CAD build for the part. Positions are in the model's coordinates, mm. Face numbers are marked on the shaded views. A direction names the side the tool comes from. Give positions to 0.01 mm unless a question says otherwise; leave off trailing zeros. Write each loop counter-clockwise with the first axis right and the second up, starting at its lowest first coordinate (ties: lowest second). Pieces come first, ordered by that corner, then holes. Notation, with made-up numbers: (41.25, -19) - (69.25, -19) arc R18 cw to (69.25, -6) - close; hole circle Ø4 at (23, 42.25). An arc over 180 degrees is marked (long way). Answer as a JSON object with one key per item and string values.
from build123d import *

# Parameters (mm, degrees)
SKETCH2_R             = 16.002
BOSS_EXTRUDE2_DEPTH   = 5.8928
CUT_EXTRUDE1_DEPTH    = 2.9464
F_4_40_TAPPED_HOLE1_D = 2.2606
CUT_EXTRUDE2_DEPTH    = 24.384890418
SKETCH5_R             = 6.35
CUT_EXTRUDE3_DEPTH    = 1.5875


with BuildPart() as part:
    # Sketch2 → Boss-Extrude2 (new body)
    with BuildSketch(Plane(origin=(0, 0, 0), x_dir=(1, 0, 0), z_dir=(0, 1, 0))):
        with Locations(Location((0, 0, 0), (0, 0, 270))):
            Circle(SKETCH2_R)
    extrude(amount=BOSS_EXTRUDE2_DEPTH)

    # Sketch2_3 → Cut-Extrude1 (cut)
    with BuildSketch(Plane(origin=(0, 0, 0), x_dir=(1, 0, 0), z_dir=(0, 1, 0))):
        with BuildLine():
            ThreePointArc((9.017, 4.192712226), (0, 9.9441), (-9.017, 4.192712226))
            Line((-9.017, 4.192712226), (-9.017, -4.192712226))
            ThreePointArc((-9.017, -4.192712226), (0, -9.9441), (9.017, -4.192712226))
            Line((9.017, -4.192712226), (9.017, 4.192712226))
        make_face()
    extrude(amount=CUT_EXTRUDE1_DEPTH, mode=Mode.SUBTRACT)

    # 4-40 Tapped Hole1 (through all)
    with Locations(Plane(origin=(-8.999982, 0, 8.999982), x_dir=(0, 0, -1), z_dir=(0, -1, 0))):
        with Locations((0, 0), (0, 17.999964), (17.999964, 17.999964), (17.999964, 0)):
            Hole(F_4_40_TAPPED_HOLE1_D / 2)

    # Sketch3 → Cut-Extrude2 (cut, through all)
    with BuildSketch(Plane.XZ):
        with BuildLine():
            ThreePointArc((3.175, 0), (1.215019898, 2.933317516), (-2.24506403, 2.24506403))
            Line((-2.24506403, 2.24506403), (2.24506403, -2.24506403))
            ThreePointArc((2.24506403, -2.24506403), (2.933317516, -1.215019898), (3.175, 0))
        make_face()
        with BuildLine():
            Line((2.24506403, -2.24506403), (-2.24506403, 2.24506403))
            ThreePointArc((-2.24506403, 2.24506403), (-2.24506403, -2.24506403), (2.24506403, -2.24506403))
        make_face()
    extrude(amount=-CUT_EXTRUDE2_DEPTH, mode=Mode.SUBTRACT)

    # Sketch5 → Cut-Extrude3 (cut)
    with BuildSketch(Plane(origin=(0, 5.8928, 0), x_dir=(1, 0, 0), z_dir=(0, 1, 0))):
        with Locations(Location((0, 0, 0), (0, 0, 270))):
            Circle(SKETCH5_R)
    extrude(amount=-CUT_EXTRUDE3_DEPTH, mode=Mode.SUBTRACT)


solid = part.part
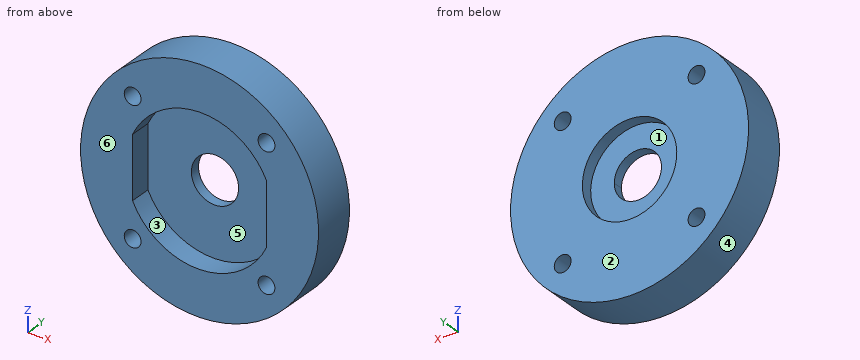
(1) Saw through at A-A, the plane x = 0. Give the cut face in (y, z) (3 decimals), and give its area (3 significant figures).
Answer key:
{"outline": "(0, -16.002) - (5.893, -16.002) - (5.893, -6.35) - (4.305, -6.35) - (4.305, -3.175) - (2.946, -3.175) - (2.946, -9.944) - (0, -9.944) - close; (0, 9.944) - (2.946, 9.944) - (2.946, 3.175) - (4.305, 3.175) - (4.305, 6.35) - (5.893, 6.35) - (5.893, 16.002) - (0, 16.002) - close", "area": "101 mm²"}
(2) Flat gauge pins, fed straight in: P1, Ø10, axis at x = 0, z = 0, coming from the -Y side; P2, Ø3, axis at x = -5.5, y = 2, coming from the -Z side; P3, Ø1, axis at x = 10.5, y = 4, coming from the +Z side. Where does each tip first touch, or does it go through?
Answer key:
{"P1": "stops at y = 2.95", "P2": "stops at z = -15.49", "P3": "stops at z = 12.49"}
(3) Saw through at C-C, the plane x = -9.5. Give the cut face in (y, z).
Answer key:
{"outline": "(0, -12.88) - (5.89, -12.88) - (5.89, -10.01) - (0, -10.01) - close; (0, -7.99) - (5.89, -7.99) - (5.89, 7.99) - (0, 7.99) - close; (0, 10.01) - (5.89, 10.01) - (5.89, 12.88) - (0, 12.88) - close"}
(4) Saw through at D-D, the plane y = 1.2. Give the cut face in (x, z).
Answer key:
{"outline": "circle Ø32 at (0, 0); hole circle Ø2.26 at (-9, -9); hole circle Ø2.26 at (-9, 9); hole (-9.02, -4.19) arc R9.94 ccw to (9.02, -4.19) - (9.02, 4.19) arc R9.94 ccw to (-9.02, 4.19) - close; hole circle Ø2.26 at (9, -9); hole circle Ø2.26 at (9, 9)"}
(5) Pull direction Z, two halves, no side cores. Call the marked faces 4, 5 and 6: pulls with the +Z half, pulls with the -Z half, needs draft (parallel to the pull), parting line crosses it, or undercut.
Answer key:
{"face 4": "parting line crosses it", "face 5": "undercut", "face 6": "needs draft"}
(6) 3-axis set-ups, long thin cutter, end or side, ignore diameter. For the marked faces 1, 2 and 3: which of +Z, -Z, +X, -X, +Y, -Y reach the whole face in a straight line?
Answer key:
{"face 1": "+Y", "face 2": "+Z, -Z, +X, -X, +Y", "face 3": "-Y"}
(7) Probe L1, parallel to X at y = 4.5, z = 8; L2, parallel to X at y = 1.1, z = -8; L3, parallel to X at y = 1.5, z = 0. List the from-to ranges inside material, lowest first. Write a range as [from, to].
Answer key:
{"L1": "x = [-13.86, -9.53], [-8.47, 8.47], [9.53, 13.86]", "L2": "x = [-13.86, -9.53], [-8.47, -5.91], [5.91, 8.47], [9.53, 13.86]", "L3": "x = [-16, -9.02], [9.02, 16]"}
(8) Saw through at B-B, the plane z = 1.5. Give the cut face in (x, y), and give its area (3 significant figures).
Answer key:
{"outline": "(-15.93, 0) - (-9.02, 0) - (-9.02, 2.95) - (-2.8, 2.95) - (-2.8, 4.31) - (-6.17, 4.31) - (-6.17, 5.89) - (-15.93, 5.89) - close; (2.8, 2.95) - (9.02, 2.95) - (9.02, 0) - (15.93, 0) - (15.93, 5.89) - (6.17, 5.89) - (6.17, 4.31) - (2.8, 4.31) - close", "area": "107 mm²"}
